Check sheet for the modelled part. Datum: model origin and axes. Units: mm. Round coordinates to 2 decimals unless told otherwise and drop trailing zeros. Order: outer loops, then holes, each group sorted by start corner. A loop starts at its lowest first (then second) coordinate and runs counter-clockwise, first axis right, second up.
(1) Sectioned sample at D-D, the plane x = 0.9. Enter the section's corners in (y, z), and give its area (3 significant figures).
(2) Mould release check, pull along Z, two halves, no side actions. Record for faces 1 (the flat face through (2, 16.25, 0)), 2 (the flat face through (1.6, 15.3, 15.2)), 3 (the cylindrical face through (0.65, -13.03, 13.15)): released by +Z, released by -Z, zero draft, split by the parting line, or undercut.
(3) Sectioned sample at B-B, the plane y = 0. Enter the section's corners in (x, z) (3 decimals).
(4) Sectioned sample at A-A, the plane z = -11.75. Enter the section's corners in (x, y) (3 decimals), and give its area (3 significant figures).
(5) Thickness scan on probe 1 along Y at (x, z) = (0.35, -11.75); probe 2 along Y at (x, z) = (0.2, 13). Record the ranges inside material, lowest first.
```python
from build123d import *

# Parameters (mm, degrees)
SKETCH1_W                                     = 32.5
SKETCH1_H                                     = 32.5
SKETCH1_R                                     = 4
BOSS_EXTRUDE1_DEPTH                           = 3.175
CHAMFER1_SIZE                                 = 2
CSK_FOR_6_FLAT_HEAD_MACHINE_SCREW1_AT_2_COUNT = 2
CSK_FOR_6_FLAT_HEAD_MACHINE_SCREW1_AT_2_PITCH = 23.5
CSK_FOR_6_FLAT_HEAD_MACHINE_SCREW1_AT_3_COUNT = 2
CSK_FOR_6_FLAT_HEAD_MACHINE_SCREW1_AT_3_PITCH = 33.234018716
CSK_FOR_6_FLAT_HEAD_MACHINE_SCREW1_AT_4_COUNT = 2
CSK_FOR_6_FLAT_HEAD_MACHINE_SCREW1_AT_4_PITCH = 23.5


with BuildPart() as part:
    # Sketch1 → Boss-Extrude1 (new body)
    with BuildSketch(Plane(origin=(0, 0, 0), x_dir=(0, 0, -1), z_dir=(1, 0, 0))):
        Rectangle(SKETCH1_W, SKETCH1_H)
        Circle(SKETCH1_R, mode=Mode.SUBTRACT)
    extrude(amount=BOSS_EXTRUDE1_DEPTH)

    # Chamfer1
    chamfer1_edges = [part.edges().sort_by_distance(p)[0] for p in [
        (1.5875, 16.25, 16.25),
        (1.5875, 16.25, -16.25),
        (1.5875, -16.25, -16.25),
        (1.5875, -16.25, 16.25),
    ]]
    chamfer(chamfer1_edges, length=CHAMFER1_SIZE)

    # Sketch3 → CSK for _6 Flat Head Machine Screw1 (revolve, cut)
    with BuildSketch(Plane(origin=(3.175, 11.75, 11.75), x_dir=(0, 0, -1), z_dir=(0, 1, 0))):
        Polygon((0, 0), (0, 3.175), (1.89865, 3.175), (1.89865, 1.891953401), (3.5433, 0), align=None)
    csk_for_6_flat_head_machine_screw1 = revolve(axis=Axis((9.525, 11.75, 11.75), (-1, 0, 0)), mode=Mode.SUBTRACT)

    # CSK for _6 Flat Head Machine Screw1 at 2: CSK for _6 Flat Head Machine Screw1 ×2
    with Locations(*[(0, 0, -i * CSK_FOR_6_FLAT_HEAD_MACHINE_SCREW1_AT_2_PITCH) for i in range(1, CSK_FOR_6_FLAT_HEAD_MACHINE_SCREW1_AT_2_COUNT)]):
        add(csk_for_6_flat_head_machine_screw1, mode=Mode.SUBTRACT)

    # CSK for _6 Flat Head Machine Screw1 at 3: CSK for _6 Flat Head Machine Screw1 ×2
    with Locations(*[Vector(0, -0.707106781, -0.707106781) * (i * CSK_FOR_6_FLAT_HEAD_MACHINE_SCREW1_AT_3_PITCH) for i in range(1, CSK_FOR_6_FLAT_HEAD_MACHINE_SCREW1_AT_3_COUNT)]):
        add(csk_for_6_flat_head_machine_screw1, mode=Mode.SUBTRACT)

    # CSK for _6 Flat Head Machine Screw1 at 4: CSK for _6 Flat Head Machine Screw1 ×2
    with Locations(*[(0, -i * CSK_FOR_6_FLAT_HEAD_MACHINE_SCREW1_AT_4_PITCH, 0) for i in range(1, CSK_FOR_6_FLAT_HEAD_MACHINE_SCREW1_AT_4_COUNT)]):
        add(csk_for_6_flat_head_machine_screw1, mode=Mode.SUBTRACT)


solid = part.part
```
Derived:
1. outline: (-16.25, -14.25) - (-14.25, -16.25) - (14.25, -16.25) - (16.25, -14.25) - (16.25, 14.25) - (14.25, 16.25) - (-14.25, 16.25) - (-16.25, 14.25) - close; hole circle Ø3.8 at (-11.75, -11.75); hole circle Ø3.8 at (-11.75, 11.75); hole circle Ø8 at (0, 0); hole circle Ø3.8 at (11.75, -11.75); hole circle Ø3.8 at (11.75, 11.75)
1. area: 953 mm2
2. face 1: zero draft
2. face 2: released by +Z
2. face 3: undercut
3. outline: (0, -16.25) - (3.175, -16.25) - (3.175, -4) - (0, -4) - close; (0, 4) - (3.175, 4) - (3.175, 16.25) - (0, 16.25) - close
4. outline: (0, -16.25) - (3.175, -16.25) - (3.175, -15.293) - (1.283, -13.649) - (0, -13.649) - close; (0, -9.851) - (1.283, -9.851) - (3.175, -8.207) - (3.175, 8.207) - (1.283, 9.851) - (0, 9.851) - close; (0, 13.649) - (1.283, 13.649) - (3.175, 15.293) - (3.175, 16.25) - (0, 16.25) - close
4. area: 72.9 mm2
5. probe 1: y = -16.25 to -13.65, -9.85 to 9.85, 13.65 to 16.25
5. probe 2: y = -16.25 to -13.18, -10.32 to 10.32, 13.18 to 16.25
